```python
from build123d import *

# Parameters (mm, degrees)
SKETCH1_W             = 63.5
SKETCH1_H             = 38.1
BOSS_EXTRUDE1_DEPTH   = 12.7
M4_CLEARANCE_HOLE1_D  = 4.5
M5X0_8_TAPPED_HOLE1_D = 4.2


with BuildPart() as part:
    # Sketch1 → Boss-Extrude1 (new body)
    with BuildSketch(Plane.XY):
        Rectangle(SKETCH1_W, SKETCH1_H)
    extrude(amount=BOSS_EXTRUDE1_DEPTH)

    # M4 Clearance Hole1 (through all)
    with Locations(Plane.XY.offset(12.7)):
        with Locations((-8, -13.05), (0, -13.05), (8, -13.05), (16, -13.05), (24, -13.05)):
            Hole(M4_CLEARANCE_HOLE1_D / 2)

    # M5x0.8 Tapped Hole1 (through all)
    with Locations(Plane.XY.offset(12.7)):
        with Locations((-20, 9.05), (-10, 9.05), (0, 9.05), (10, 9.05)):
            Hole(M5X0_8_TAPPED_HOLE1_D / 2)


solid = part.part
```
Could you check a few things on this model? Use its own coordinates, in mm. Round coordinates to 2 decimals unless told otherwise and drop trailing zeros. Loops run counter-clockwise (first coordinate to the right, second up) from the corner with the lowest first, then second, coordinate; pieces in that order, holes last. Notation, with made-up numbers: M 64.25,-30 L 71.25,-30 A20 cw 71.25,1 Z; hole C 3,-17.5 d8. An arc over 180 degrees is marked long. Write item = value, one per line.
1. I need wall thicknesses on probe 1 along Y at (x, z) = (0, 6.75); probe 2 along X at (y, z) = (9, 11); probe 3 along Y at (x, z) = (24, 9.75). Which ranges of each line are inside material? Lowest first, please.
Results below:
probe_1 = -19.05 to -15.3, -10.8 to 6.95, 11.15 to 19.05
probe_2 = -31.75 to -22.1, -17.9 to -12.1, -7.9 to -2.1, 2.1 to 7.9, 12.1 to 31.75
probe_3 = -19.05 to -15.3, -10.8 to 19.05
2. Thinking about a two-plate mould opening in X: for faces 1 (the face through (0.46, 7, 6.26)), 2 (the face through (0, -19.05, 6)), 3 (the face through (31.75, 0, 6)), which applies, +X half, -X half, draft (parallel to the pull), parting line (faces both ways), or undercut?
Results below:
face_1 = undercut
face_2 = draft
face_3 = +X half
3. I want a section at B-B, the plane y = 9.05. Write out the boundary of the cut face in (x, z).
Results below:
outline = M -31.75,0 L -22.1,0 L -22.1,12.7 L -31.75,12.7 Z; M -17.9,0 L -12.1,0 L -12.1,12.7 L -17.9,12.7 Z; M -7.9,0 L -2.1,0 L -2.1,12.7 L -7.9,12.7 Z; M 2.1,0 L 7.9,0 L 7.9,12.7 L 2.1,12.7 Z; M 12.1,0 L 31.75,0 L 31.75,12.7 L 12.1,12.7 Z
4. I want a section at C-C, the plane x = 16. Write out the boundary of the cut face in (y, z), and give its area (3 significant figures).
Results below:
outline = M -19.05,0 L -15.3,0 L -15.3,12.7 L -19.05,12.7 Z; M -10.8,0 L 19.05,0 L 19.05,12.7 L -10.8,12.7 Z
area = 427 mm²
5. I want a section at D-D, the plane z = 9.75. Count the separate pieces of the cut face and the enclosed holes in it, and give its area (3 significant figures).
Results below:
separate_pieces = 1
enclosed_holes = 9
area = 2,280 mm²
6. Will these pins go through, and if not, where does the flat tip stop? P1, Ø4, axis at x = 0, y = -13.05, coming from the +Z side; P2, Ø6.5, axis at x = -10, y = 9.05, coming from the +Z side.
Results below:
P1 = through
P2 = 12.7
7. I want a section at A-A, the plane x = 0. Write out the boundary of the cut face in (y, z).
Results below:
outline = M -19.05,0 L -15.3,0 L -15.3,12.7 L -19.05,12.7 Z; M -10.8,0 L 6.95,0 L 6.95,12.7 L -10.8,12.7 Z; M 11.15,0 L 19.05,0 L 19.05,12.7 L 11.15,12.7 Z
